Model file for the job. Use its own axes, mm. Give positions to 0.01 mm unless a question says otherwise; leave off trailing zeros. Order: outer loops, then holes, each group sorted by start corner. A loop starts at its lowest first (then second) coordinate and runs counter-clockwise, first axis right, second up. Notation, with made-up numbers: M 88.5,59.25 L 136.5,59.25 A23 cw 136.5,74.25 Z; hole C 73.25,85.5 d2. An arc over 180 degrees is marked long. Return JSON: item names as keys, results as strings. Group by question number.
1. Slice it at A-A on x = 0. List the corners of the cut face in (y, z) (3 decimals).
2. Slice it at D-D on x = -18.5. List the corners of the cut face in (y, z), then the cut area to 3 significant figures.
3. Wall check: probe 1 along Y at (x, z) = (-0.5, 9.75); probe 2 along X at (y, z) = (2, 2.75); probe 3 along X at (y, z) = (-6, 11). Give the ranges that are in metal, low to high. Write a range as [from, to].
4. Two-plate mould, pull along X, no slides. Class faces 1 (the face through (0, -14, 0)), 2 (the face through (-15.618, -10.683, 14.79)), 3 (the face through (-2.17, -9.76, 14.79)): released by +X, released by -X, zero draft, split by the parting line, or undercut.
5. Slice it at B-B on z = 23.75. List the corners of the cut face in (x, y) (3 decimals).
6. Pin check, flat tips, straight feed: pin 1 (1.5 mm diameter, centred on y = 4.5, z = 15.5, fed in from -X); pin 2 (5 mm diameter, centred on y = -3, z = 26.5, fed in from +X); pin 3 (10 mm diameter, centred on y = -4.5, z = 23.5, fed in from +X). Stop position of each tip, or through.
7. Slice it at C-C on y = -7.5. List the corners of the cut face in (x, z).
from build123d import *

# Parameters (mm, degrees)
SKETCH1_R           = 10
BOSS_EXTRUDE1_DEPTH = 30


with BuildPart() as part:
    # Sketch1 → Boss-Extrude1 (new body)
    with BuildSketch(Plane.XY):
        with BuildLine():
            ThreePointArc((13.175, 0), (15.552506488, -10.54520033), (22.225, -19.05))
            Line((22.225, -19.05), (22.225, -25.4))
            Line((22.225, -25.4), (-22.225, -25.4))
            Line((-22.225, -25.4), (-22.225, -19.05))
            ThreePointArc((-22.225, -19.05), (-15.552506488, -10.54520033), (-13.175, 0))
            ThreePointArc((-13.175, 0), (0, 13.175), (13.175, 0))
        make_face()
        Circle(SKETCH1_R, mode=Mode.SUBTRACT)
    extrude(amount=BOSS_EXTRUDE1_DEPTH)


solid = part.part
Result:
{
 "1": {"outline": "M -25.4,0 L -10,0 L -10,30 L -25.4,30 Z; M 10,0 L 13.175,0 L 13.175,30 L 10,30 Z"},
 "2": {"outline": "M -25.4,0 L -15.28,0 L -15.28,30 L -25.4,30 Z", "area": "304 mm2"},
 "3": {"probe 1": "y = [-25.4, -9.99], [9.99, 13.17]", "probe 2": "x = [-13.02, -9.8], [9.8, 13.02]", "probe 3": "x = [-13.92, -8], [8, 13.92]"},
 "4": {"face 1": "zero draft", "face 2": "released by -X", "face 3": "undercut"},
 "5": {"outline": "M -22.225,-25.4 L 22.225,-25.4 L 22.225,-19.05 A24.575 cw 13.175,0 A13.175 ccw -13.175,0 A24.575 cw -22.225,-19.05 Z; hole C 0,0 d20"},
 "6": {"pin 1": "stops at x = -12.63", "pin 2": "stops at x = 13.8", "pin 3": "stops at x = 15.09"},
 "7": {"outline": "M -14.35,0 L -6.61,0 L -6.61,30 L -14.35,30 Z; M 6.61,0 L 14.35,0 L 14.35,30 L 6.61,30 Z"}
}
